Geometry: final body of the model. Coordinates: model frame, mm. Give positions to 0.01 mm unless a question says otherwise; leave off trailing zeros. Write each loop counter-clockwise with the first axis right and the second up, starting at its lowest first coordinate (ties: lowest second). Pieces come first, ordered by that corner, then holes. Notation, with made-up numbers: (45.5, 73) - (69.5, 73) arc R12 ccw to (69.5, 87) - close; hole circle Ø11 at (-9.5, 15.5). An arc over 180 degrees is marked (long way). Return JSON: item names as keys, results as strings.
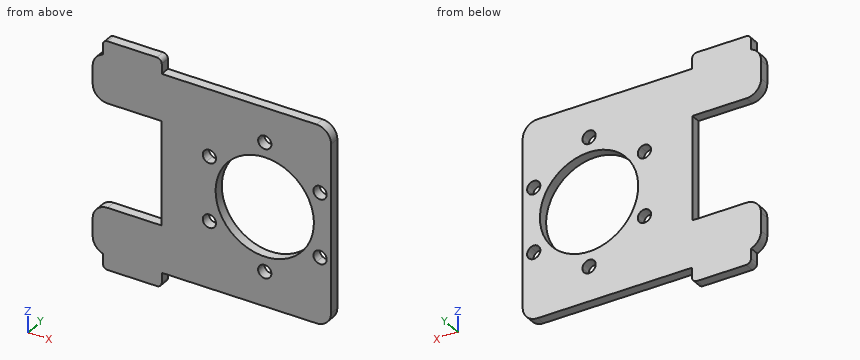
from build123d import *

# Parameters (mm, degrees)
SKETCH_1_W      = 12
SKETCH_1_H      = 3
SKETCH_1_R      = 10
EXTRUDE_1_DEPTH = 2
FILLET_1_R      = 3
FILLET_2_R      = 1


with BuildPart() as part:
    # 草图1 → 凸台-拉伸1 (new body)
    # profile 1 of 4: a face of its own
    with BuildSketch(Plane(origin=(0, 0, 0), x_dir=(1, 0, 0), z_dir=(0, 1, 0))):
        Polygon((-24.25, -10.5), (-24.25, -20), (-22.2, -20), (-10.2, -20), (24.25, -20), (24.25, 20), (-10.2, 20), (-22.2, 20), (-24.25, 20), (-24.25, 10.5), (-10.25, 10.5), (-10.25, -10.5), align=None)
        with BuildLine():
            ThreePointArc((22.621714683, 5.297394688), (23.75, 0), (22.621714683, -5.297394688))
            ThreePointArc((22.621714683, -5.297394688), (23.159540262, -5.794864902), (23.358330249, -6.5))
            ThreePointArc((23.358330249, -6.5), (22.652739816, -7.686269915), (21.273535715, -7.632509158))
            ThreePointArc((21.273535715, -7.632509158), (17.25, -11.258330249), (12.098178968, -12.929903846))
            ThreePointArc((12.098178968, -12.929903846), (12.099544665, -12.964940098), (12.1, -13))
            ThreePointArc((12.1, -13), (10.714940098, -14.349544665), (9.401821032, -12.929903846))
            ThreePointArc((9.401821032, -12.929903846), (4.25, -11.258330249), (0.226464285, -7.632509158))
            ThreePointArc((0.226464285, -7.632509158), (-1.677464544, -7.175), (-1.121714683, -5.297394688))
            ThreePointArc((-1.121714683, -5.297394688), (-2.25, 0), (-1.121714683, 5.297394688))
            ThreePointArc((-1.121714683, 5.297394688), (-1.677464544, 7.175), (0.226464285, 7.632509158))
            ThreePointArc((0.226464285, 7.632509158), (4.25, 11.258330249), (9.401821032, 12.929903846))
            ThreePointArc((9.401821032, 12.929903846), (10.714940098, 14.349544665), (12.1, 13))
            ThreePointArc((12.1, 13), (12.099544665, 12.964940098), (12.098178968, 12.929903846))
            ThreePointArc((12.098178968, 12.929903846), (17.25, 11.258330249), (21.273535715, 7.632509158))
            ThreePointArc((21.273535715, 7.632509158), (22.652739816, 7.686269915), (23.358330249, 6.5))
            ThreePointArc((23.358330249, 6.5), (23.159540262, 5.794864902), (22.621714683, 5.297394688))
        make_face(mode=Mode.SUBTRACT)
    # profile 2 of 4: a face of its own
    with BuildSketch(Plane(origin=(0, 0, 0), x_dir=(1, 0, 0), z_dir=(0, 1, 0))):
        with Locations((-16.2, 21.5)):
            Rectangle(SKETCH_1_W, SKETCH_1_H)
    # profile 3 of 4: a face of its own
    with BuildSketch(Plane(origin=(0, 0, 0), x_dir=(1, 0, 0), z_dir=(0, 1, 0))):
        with Locations((-16.2, -21.5)):
            Rectangle(SKETCH_1_W, SKETCH_1_H)
    # profile 4 of 4: a face of its own
    with BuildSketch(Plane(origin=(0, 0, 0), x_dir=(1, 0, 0), z_dir=(0, 1, 0))):
        with BuildLine():
            ThreePointArc((21.273535715, -7.632509158), (20.839195954, -5.825), (22.621714683, -5.297394688))
            ThreePointArc((22.621714683, -5.297394688), (23.75, 0), (22.621714683, 5.297394688))
            ThreePointArc((22.621714683, 5.297394688), (20.839195954, 5.825), (21.273535715, 7.632509158))
            ThreePointArc((21.273535715, 7.632509158), (17.25, 11.258330249), (12.098178968, 12.929903846))
            ThreePointArc((12.098178968, 12.929903846), (10.75, 11.65), (9.401821032, 12.929903846))
            ThreePointArc((9.401821032, 12.929903846), (4.25, 11.258330249), (0.226464285, 7.632509158))
            ThreePointArc((0.226464285, 7.632509158), (0.677939665, 7.144409567), (0.841669751, 6.5))
            ThreePointArc((0.841669751, 6.5), (0.196804849, 5.348789987), (-1.121714683, 5.297394688))
            ThreePointArc((-1.121714683, 5.297394688), (-2.25, 0), (-1.121714683, -5.297394688))
            ThreePointArc((-1.121714683, -5.297394688), (0.196804849, -5.348789987), (0.841669751, -6.5))
            ThreePointArc((0.841669751, -6.5), (0.677939665, -7.144409567), (0.226464285, -7.632509158))
            ThreePointArc((0.226464285, -7.632509158), (4.25, -11.258330249), (9.401821032, -12.929903846))
            ThreePointArc((9.401821032, -12.929903846), (10.75, -11.65), (12.098178968, -12.929903846))
            ThreePointArc((12.098178968, -12.929903846), (17.25, -11.258330249), (21.273535715, -7.632509158))
        make_face()
        with Locations(Location((10.75, 0, 0), (0, 0, 270))):
            Circle(SKETCH_1_R, mode=Mode.SUBTRACT)
    extrude(amount=EXTRUDE_1_DEPTH)

    # 圆角1
    # the kernel refuses this fillet: 3 mm, written as the material it takes off along each edge
    with BuildSketch(Plane(origin=(-24.25, -7.5, -10.5), x_dir=(1, 0, 0), z_dir=(0, 1, 0)), Plane(origin=(24.25, -7.5, -20), x_dir=(-1, 0, 0), z_dir=(0, 1, 0)), Plane(origin=(24.25, -7.5, 20), x_dir=(0, 0, -1), z_dir=(0, 1, 0)), Plane(origin=(-24.25, -7.5, 10.5), x_dir=(0, 0, 1), z_dir=(0, 1, 0))) as fillet_1_piece_1:
        with BuildLine():
            CenterArc((FILLET_1_R, FILLET_1_R), FILLET_1_R, 180, 90)
            Line((0, FILLET_1_R), (-FILLET_1_R * 0.02, FILLET_1_R))
            Line((-FILLET_1_R * 0.02, FILLET_1_R), (-FILLET_1_R * 0.02, -FILLET_1_R * 0.02))
            Line((-FILLET_1_R * 0.02, -FILLET_1_R * 0.02), (FILLET_1_R, -FILLET_1_R * 0.02))
            Line((FILLET_1_R, -FILLET_1_R * 0.02), (FILLET_1_R, 0))
        make_face()
    extrude(amount=17, mode=Mode.SUBTRACT)
    with BuildSketch(Plane(origin=(-24.25, -7.114026638, -20), x_dir=(0, 0, 1), z_dir=(0, 1, 0))) as fillet_1_piece_2:
        with BuildLine():
            CenterArc((2.845610655, 3), FILLET_1_R, 198.461458297, 71.538541703)
            Line((0, 2.05), (-0.056912213, 2.031))
            ThreePointArc((-0.056912213, 2.031), (-0.06, 1.025), (-0.06, 0))
            Line((-0.06, 0), (0, -0.06))
            Line((0, -0.06), (2.845610655, -0.06))
            Line((2.845610655, -0.06), (2.845610655, 0))
        make_face()
    extrude(amount=16.228053275, mode=Mode.SUBTRACT)
    with BuildSketch(Plane(origin=(-24.25, -7.114026638, 20), x_dir=(0, 0, -1), z_dir=(0, 1, 0))) as fillet_1_piece_3:
        with BuildLine():
            CenterArc((2.845610655, -3), FILLET_1_R, 90, 71.538541703)
            Line((0, -2.05), (-0.056912213, -2.031))
            ThreePointArc((-0.056912213, -2.031), (-0.06, -1.025), (-0.06, 0))
            Line((-0.06, 0), (0, 0.06))
            Line((0, 0.06), (2.845610655, 0.06))
            Line((2.845610655, 0.06), (2.845610655, 0))
        make_face()
    extrude(amount=16.228053275, mode=Mode.SUBTRACT)

    # 圆角2
    fillet_2_edges = [part.edges().sort_by_distance(p)[0] for p in [
        (-22.2, 1, -23),
        (-10.2, 1, -23),
        (-10.2, 1, 23),
        (-22.2, 1, 23),
    ]]
    fillet(fillet_2_edges, radius=FILLET_2_R)


solid = part.part
Q1. Pin query (flat end, axial travel): P1, Ø1, axis at y = 0.5, z = -0.5, coming from the -X side; P2, Ø1, axis at x = 11, y = 1, coming from the +Z side; P3, Ø0.6, axis at y = 0.5, z = -21, coming from the -X side; P4, Ø6, axis at x = -14.5, z = 5, coming from the -Y side. Return the tip coordinate at first contact, or that it passes through.
Answer key:
{"P1": "stops at x = -10.25", "P2": "stops at z = 20", "P3": "stops at x = -22.2", "P4": "passes through"}
Q2. Material intervals for probe 1 along X at (y, z) = (1.25, 0); probe 2 along X at (y, z) = (0.55, -5.5); probe 3 along Z at (x, y) = (-7, 0.75), sorted ascending. Write a range as [from, to].
Answer key:
{"probe 1": "x = [-10.25, 0.75], [20.75, 24.25]", "probe 2": "x = [-10.25, -1.42], [0.4, 2.4], [19.1, 21.1], [22.92, 24.25]", "probe 3": "z = [-20, 20]"}
Q3. Section query D-D, the plane y = 1.2. Count the separate pieces of the cut face and the enclosed holes in it, plus the area to 3 significant figures.
Answer key:
{"separate pieces": "1", "enclosed holes": "7", "area": "1,360 mm^2"}
Q4. Section query A-A, the plane z = 0. Return the cut outline in (x, y), plus the area to 3 significant figures.
Answer key:
{"outline": "(-10.25, 0) - (0.75, 0) - (0.75, 2) - (-10.25, 2) - close; (20.75, 0) - (24.25, 0) - (24.25, 2) - (20.75, 2) - close", "area": "29.0 mm^2"}
Q5. Section query B-B, the plane x = 10.75. Return the cut outline in (y, z).
Answer key:
{"outline": "(0, -20) - (2, -20) - (2, -14.35) - (0, -14.35) - close; (0, -11.65) - (2, -11.65) - (2, -10) - (0, -10) - close; (0, 10) - (2, 10) - (2, 11.65) - (0, 11.65) - close; (0, 14.35) - (2, 14.35) - (2, 20) - (0, 20) - close"}
Q6. Section query C-C, the plane x = -0.5. Return the cut outline in (y, z), plus the area to 3 significant figures.
Answer key:
{"outline": "(0, -20) - (2, -20) - (2, -7.85) - (0, -7.85) - close; (0, -5.15) - (2, -5.15) - (2, 5.15) - (0, 5.15) - close; (0, 7.85) - (2, 7.85) - (2, 20) - (0, 20) - close", "area": "69.2 mm^2"}
